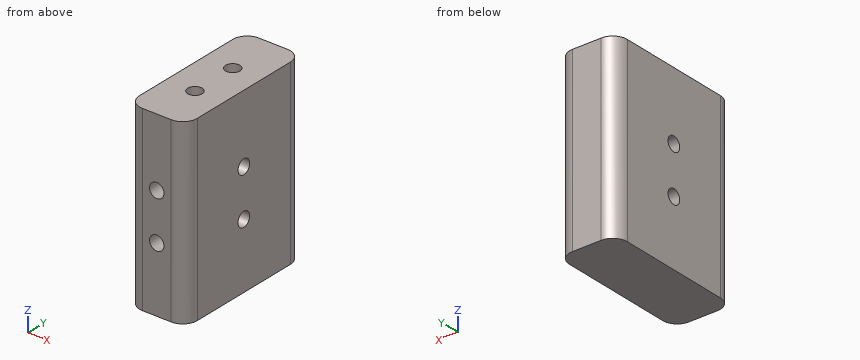
```python
from build123d import *

# Parameters (mm, degrees)
F0_W     = 20
F0_H     = 25
F1_DEPTH = 4
F2_R     = 1
F5_DEPTH = 25
F3_R     = 1
F6_DEPTH = 5
F4_R     = 1
F7_DEPTH = 5
F8_R     = 2


with BuildPart() as f1:
    # F0 (on Right) → F1 (new body, symmetric)
    with BuildSketch(Plane.YZ):
        Rectangle(F0_W, F0_H)
    extrude(amount=F1_DEPTH, both=True)

    # F2 (on face) → F5 (cut)
    with BuildSketch(Plane.YZ.offset(4)):
        with Locations((0, 3.05)):
            Circle(F2_R)
        with Locations((0, -3.45)):
            Circle(F2_R)
    extrude(amount=-F5_DEPTH, mode=Mode.SUBTRACT)

    # F3 (on face) → F6 (cut)
    with BuildSketch(Plane.XY.offset(12.5)):
        with Locations((0, -3.45)):
            Circle(F3_R)
        with Locations((0, 3.05)):
            Circle(F3_R)
    extrude(amount=-F6_DEPTH, mode=Mode.SUBTRACT)

    # F4 (on face) → F7 (cut)
    with BuildSketch(Plane.XZ.offset(10)):
        with Locations((0, 3.05)):
            Circle(F4_R)
        with Locations((0, -3.45)):
            Circle(F4_R)
    extrude(amount=-F7_DEPTH, mode=Mode.SUBTRACT)

    # F8
    f8_edges = [f1.edges().sort_by_distance(p)[0] for p in [
        (4, -10, 0),
        (-4, -10, 0),
        (4, 10, 0),
        (-4, 10, 0),
    ]]
    fillet(f8_edges, radius=F8_R)


solid = f1.part
```
The model under review builds one solid part; all positions refer to its coordinate system, in mm. Round coordinates to 2 decimals unless told otherwise and drop trailing zeros. Write each loop counter-clockwise with the first axis right and the second up, starting at its lowest first coordinate (ties: lowest second). Pieces come first, ordered by that corner, then holes. Notation, with made-up numbers: (15.5, 36) - (42.5, 36) arc R6 ccw to (42.5, 43) - close; hole circle Ø3 at (-19, 65.5). An arc over 180 degrees is marked (long way). Answer as CSV lines item,"result". Start each with the question number.
(1) We need section C-C on x = 0. State the section outline as (y, z) points, plus the area to 3 significant figures.
(2) We need section D-D on z = 10.75. State the section outline as (x, y) points.
(3) We need section B-B on y = 0. State the section outline as (x, z) points.
(4) For pin 1 Ø2.5 at (y, z) = (0, 3.05) entering from -X; pin 2 Ø1.6 at (x, y) = (0, -3.45) entering from +Z; pin 3 Ø1.2 at (y, z) = (0, -3.45) entering from +X; pin 4 Ø1.8 at (x, z) = (0, -3.45) entering from -Y, all flat-tipped, find the tip position at first contact; note any pin that passes through.
(5) We need section A-A on z = -3.45. State the section outline as (x, y) points.
(6) To check wall thickness, follow line 1 (Z direction, x = 0, y = -7.5); line 2 (Y direction, x = 0, z = 9.8); line 3 (X direction, y = -8, z = -4.25). State the ranges of each line that lie inside material, in increasing order.
Worked answers:
1,outline,"(-10, -12.5) - (10, -12.5) - (10, 12.5) - (4.05, 12.5) - (4.05, 7.5) - (2.05, 7.5) - (2.05, 12.5) - (-2.45, 12.5) - (-2.45, 7.5) - (-4.45, 7.5) - (-4.45, 12.5) - (-10, 12.5) - (-10, 4.05) - (-5, 4.05) - (-5, 2.05) - (-10, 2.05) - (-10, -2.45) - (-5, -2.45) - (-5, -4.45) - (-10, -4.45) - close; hole circle Ø2 at (0, -3.45); hole circle Ø2 at (0, 3.05)"
1,area,"454 mm²"
2,outline,"(-4, -8) arc R2 ccw to (-2, -10) - (2, -10) arc R2 ccw to (4, -8) - (4, 8) arc R2 ccw to (2, 10) - (-2, 10) arc R2 ccw to (-4, 8) - close; hole circle Ø2 at (0, -3.45); hole circle Ø2 at (0, 3.05)"
3,outline,"(-4, -12.5) - (4, -12.5) - (4, -4.45) - (-4, -4.45) - close; (-4, -2.45) - (4, -2.45) - (4, 2.05) - (-4, 2.05) - close; (-4, 4.05) - (4, 4.05) - (4, 12.5) - (-4, 12.5) - close"
4,pin 1,"x = -4"
4,pin 2,"z = 7.5"
4,pin 3,"through"
4,pin 4,"y = -5"
5,outline,"(-4, -8) arc R2 ccw to (-2, -10) - (-1, -10) - (-1, -5) - (1, -5) - (1, -10) - (2, -10) arc R2 ccw to (4, -8) - (4, -1) - (-4, -1) - close; (-4, 1) - (4, 1) - (4, 8) arc R2 ccw to (2, 10) - (-2, 10) arc R2 ccw to (-4, 8) - close"
6,line 1,"-12.5 to -4.45, -2.45 to 2.05, 4.05 to 12.5"
6,line 2,"-10 to -4.45, -2.45 to 2.05, 4.05 to 10"
6,line 3,"-4 to -0.6, 0.6 to 4"
